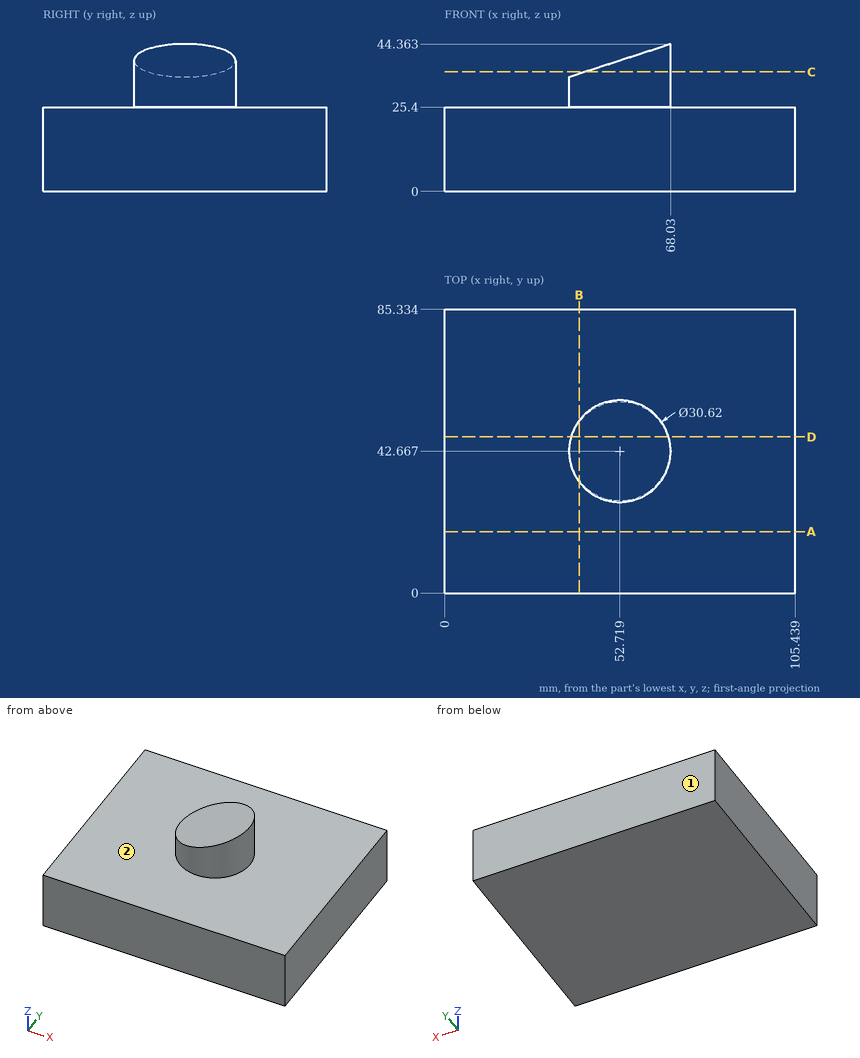
Check sheet for the drawn part. Datum: minimum x, y, z corner. Units: mm. A direction names the side the tool comes from. Give positions to 0.01 mm unless a question says otherwise; leave off trailing zeros. Order: outer loops, then holes, each group sorted by start corner. A loop starts at its lowest first (then second) coordinate and runs counter-clockwise, first axis right, second up. Notation, with made-up numbers: (58.25, 30) -> (106.25, 30) arc R30 cw to (106.25, 63) -> close; hole circle Ø10 at (-28.75, 70.25). An arc over 180 degrees is marked (long way). Return JSON: item names as keys, results as strings.
1. Go/stop test with flat-tipped pins: P1, Ø10, axis at y = 48.5, z = 33, coming from the -X side; P2, Ø4, axis at x = 41.5, y = 70.5, coming from the +Z side; P3, Ø5, axis at x = 21.5, y = 56, coming from the -Z side; P4, Ø8, axis at x = 52.5, z = 36.5, coming from the +Y side. Record where each tip stops, or that it passes through.
From the geometry:
{"P1": "x = 37.43", "P2": "z = 25.4", "P3": "z = 0", "P4": "y = 57.98"}
2. Cross-section at A-A, the plane y = 18.5. Record the cut outline in (x, z).
From the geometry:
{"outline": "(0, 0) -> (105.44, 0) -> (105.44, 25.4) -> (0, 25.4) -> close"}
3. Cross-section at D-D, the plane y = 47. Record the cut outline in (x, z) (1 decimal).
From the geometry:
{"outline": "(0, 0) -> (105.4, 0) -> (105.4, 25.4) -> (67.4, 25.4) -> (67.4, 44.2) -> (38, 34.6) -> (38, 25.4) -> (0, 25.4) -> close"}
4. Set-up check for the marked faces 1 and 2: record each of +Z, -Z, +X, -X, +Y, -Y from which the full face is reachable in a straight line by a thin tool's end or side.
From the geometry:
{"face 1": "+Z, -Z, +X, -X, +Y", "face 2": "+Z"}
5. Material ranges on probe 1 along Z at (x, y) = (44, 81.5); probe 2 along X at (y, z) = (56, 30.5) (1 decimal); probe 3 along Z at (x, y) = (44, 47.5) (1 decimal), recorded low to high. Write a range as [from, to].
From the geometry:
{"probe 1": "[0, 25.4]", "probe 2": "[45.2, 60.2]", "probe 3": "[0, 36.6]"}
6. Cross-section at C-C, the plane z = 36. Record the cut outline in (x, y) (1 decimal).
From the geometry:
{"outline": "(42.3, 31.5) arc R15.3 ccw (long way) to (42.3, 53.8) -> close"}
7. Cross-section at B-B, the plane x = 40.5. Record the cut outline in (y, z) (1 decimal), plus the area to 3 significant figures.
From the geometry:
{"outline": "(0, 0) -> (85.3, 0) -> (85.3, 25.4) -> (51.9, 25.4) -> (51.9, 35.4) -> (33.4, 35.4) -> (33.4, 25.4) -> (0, 25.4) -> close", "area": "2,350 mm^2"}
